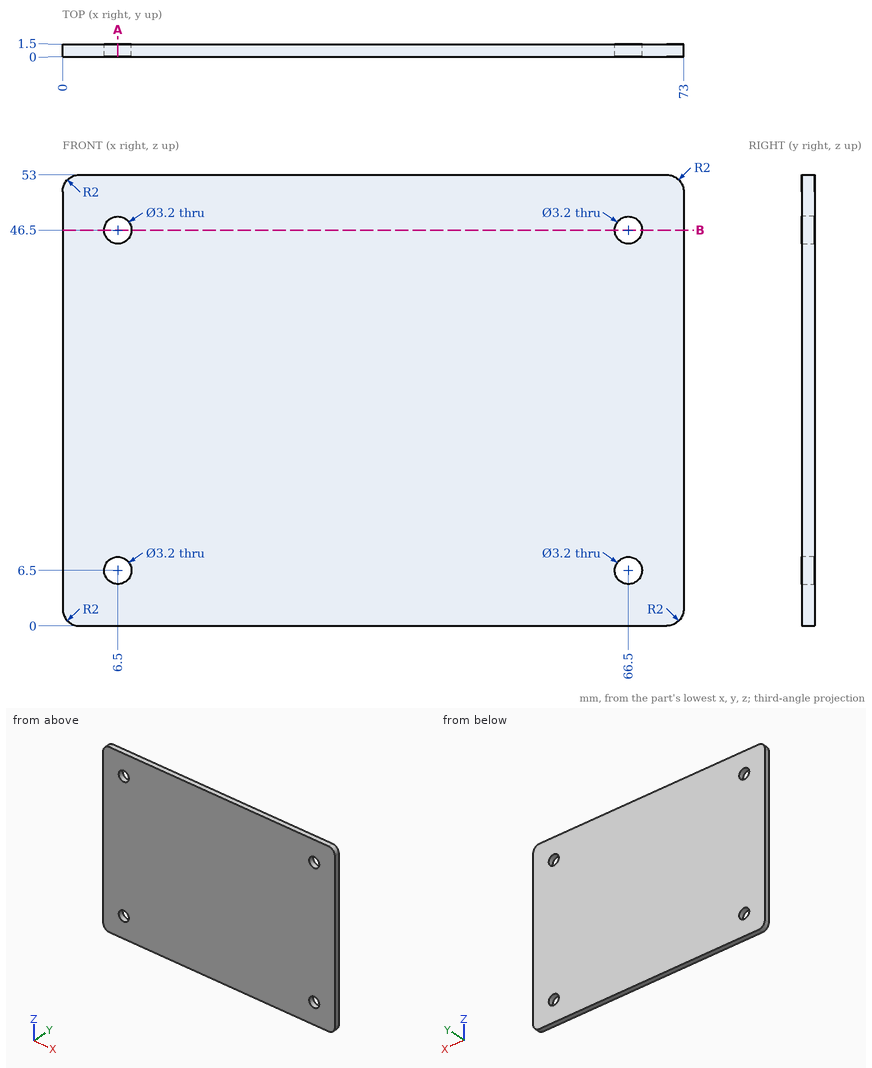
Input: dimensioned drawing with shaded views. Units: mm. Origin: part minimum x, y, z. Give positions to 0.01 mm unless a question says otherwise; leave off trailing zeros. Loops run counter-clockwise (first coordinate to the right, second up) from the corner with the lowest first, then second, coordinate; pieces in that order, holes last. Notation, with made-up numbers: (88.5, 45.5) -> (92.5, 45.5) arc R13 cw to (92.5, 70.5) -> close; hole circle Ø10 at (-35.75, 23.25). An arc over 180 degrees is marked (long way). Use a Markdown table: item, result.
Q1. Section query B-B, the plane z = 46.5. Return the cut outline in (x, y).
Entries:
| item | result |
|---|---|
| outline | (0, 0) -> (4.9, 0) -> (4.9, 1.5) -> (0, 1.5) -> close; (8.1, 0) -> (64.9, 0) -> (64.9, 1.5) -> (8.1, 1.5) -> close; (68.1, 0) -> (73, 0) -> (73, 1.5) -> (68.1, 1.5) -> close |
Q2. First-contact query: P1, Ø5, axis at x = 6.5, z = 6.5, coming from the -Y side. Flat tip, straight axial feed; report the tip coordinate or a pass-through.
Entries:
| item | result |
|---|---|
| P1 | stops at y = 0 |
Q3. Section query A-A, the plane x = 6.5. Return the cut outline in (y, z).
Entries:
| item | result |
|---|---|
| outline | (0, 0) -> (1.5, 0) -> (1.5, 4.9) -> (0, 4.9) -> close; (0, 8.1) -> (1.5, 8.1) -> (1.5, 44.9) -> (0, 44.9) -> close; (0, 48.1) -> (1.5, 48.1) -> (1.5, 53) -> (0, 53) -> close |
Q4. Ray query, probe 1 along X at (y, z) = (0.6, 6.5); probe 2 along X at (y, z) = (0.9, 47). Return the intervals inside material, ascending. Write a range as from..to.
Entries:
| item | result |
|---|---|
| probe 1 | x = 0..4.9, 8.1..64.9, 68.1..73 |
| probe 2 | x = 0..4.98, 8.02..64.98, 68.02..73 |
